For this review, take the finished solid that the model builds, in its own axes (mm). A direction names the side the tool comes from. Round coordinates to 2 decimals unless told otherwise and drop trailing zeros. Write each loop counter-clockwise with the first axis right and the second up, starting at its lowest first coordinate (ties: lowest second). Pieces come first, ordered by that corner, then holes. Notation, with made-up numbers: M 50,-22 L 80,-22 A29 ccw 80,4 Z; hole C -9.75,-15.75 d4. An arc over 180 degrees is marked long. Use one line per item in the form item = value. Start each with the question number.
Item 1: Add section A-A (x = 5.5). State the section outline as (y, z) points.
Item 2: For P1, Ø8.5, axis at x = -5, z = 4, coming from the +Y side; P2, Ø3, axis at y = 4.5, z = 3, coming from the +X side; P3, Ø3, axis at x = -8, z = -6, coming from the +Y side, all flat-tipped, find the tip position at first contact; note any pin that passes through.
Item 3: Draft analysis for pull direction Z (two halves, no side actions). For faces 1 (the conical face through (1.35, 3.288, 1.375)), 2 (the flat face through (5, 0.5, -4)), 3 (the flat face through (0, 0, 0)), 4 (the conical face through (-10.4, 3, 8.3)), state which applies: released by +Z, released by -Z, zero draft, split by the parting line, or undercut.
Item 4: Add section B-B (z = 4). State the section outline as (x, y) points, and give its area (3 significant figures).
Item 5: For line 1 (Z direction, x = 5.75, y = 1.25); line 2 (X direction, y = 1, z = 5.5); line 3 (Y direction, x = -9, z = -7), list the stretches that pass through material, from the lowest coordinate up. Write a range as [from, to].
Item 6: For faces 5 (the conical face through (10.21, 0.99, 8.23)), 6 (the conical face through (10.3, 3, 8.4)), 7 (the flat face through (10.704, 2.986, -0.105)), 8 (the conical face through (-10.23, 0.99, 8.21)), 9 (the conical face through (-0.218, 3.288, -1.663)), list the 3-axis set-ups (+Z, -Z, +X, -X, +Y, -Y) from which the entire face can be reached by the end or side of a thin tool; tool diameter is ignored.
from build123d import *

# Parameters (mm, degrees)
BOSS_EXTRUDE1_DEPTH = 4
BOSS_EXTRUDE1_DRAFT = -1
SHELL1_T            = -0.5
SKETCH2_R           = 2
BOSS_EXTRUDE2_DEPTH = 5.5
BOSS_EXTRUDE2_TAPER = 1.5
CIRPATTERN1_COUNT   = 4
SKETCH4_R           = 1.605977431
CUT_EXTRUDE1_DEPTH  = 5.5
CUT_EXTRUDE1_DRAFT  = 1.5
RIB2_START          = -10.069744096
RIB2_DEPTH          = 8.231928651
RIB2_START_2        = 1.837815445
RIB2_2_DEPTH        = 8.231928651
RIB2_START_3        = -8.069744096
RIB2_3_DEPTH        = 6.231928651
RIB2_4_DEPTH        = 6.231928651


with BuildPart() as part:
    # Sketch1 → Boss-Extrude1 (with draft: the straight prism first)
    with BuildSketch(Plane(origin=(0, 0, 0), x_dir=(1, 0, 0), z_dir=(0, 1, 0))):
        with BuildLine():
            Line((-9.5, -8.5), (9.5, -8.5))
            ThreePointArc((9.5, -8.5), (10.207106781, -8.207106781), (10.5, -7.5))
            Line((10.5, -7.5), (10.5, 7.5))
            ThreePointArc((10.5, 7.5), (10.207106781, 8.207106781), (9.5, 8.5))
            Line((9.5, 8.5), (-9.5, 8.5))
            ThreePointArc((-9.5, 8.5), (-10.207106781, 8.207106781), (-10.5, 7.5))
            Line((-10.5, 7.5), (-10.5, -7.5))
            ThreePointArc((-10.5, -7.5), (-10.207106781, -8.207106781), (-9.5, -8.5))
        make_face()
    extrude(amount=BOSS_EXTRUDE1_DEPTH)
    # Boss-Extrude1: the draft: its side faces are tilted about the plane it starts from
    boss_extrude1_sides = [part.faces().sort_by_distance(p)[0] for p in [
        (0, 2, 8.5),
        (10.207106781, 2, 8.207106781),
        (10.5, 2, 0),
        (10.207106781, 2, -8.207106781),
        (0, 2, -8.5),
        (-10.207106781, 2, -8.207106781),
        (-10.5, 2, 0),
        (-10.207106781, 2, 8.207106781),
    ]]
    draft(boss_extrude1_sides, Plane(origin=(0, 0, 0), x_dir=(1, 0, 0), z_dir=(0, 1, 0)), BOSS_EXTRUDE1_DRAFT)

    # Shell1
    shell1_openings = [part.faces().sort_by_distance(p)[0] for p in [
        (0, 4, 0),
    ]]
    offset(amount=SHELL1_T, openings=shell1_openings, kind=Kind.INTERSECTION)

    # Sketch2 → Boss-Extrude2 (add)
    with BuildSketch(Plane(origin=(0, 0.5, 0), x_dir=(1, 0, 0), z_dir=(0, 1, 0))):
        Circle(SKETCH2_R)
    extrude(amount=BOSS_EXTRUDE2_DEPTH, taper=BOSS_EXTRUDE2_TAPER)

    # Rib1: read off the stored shape, not the designer's step
    # Rib1: loft between two sections, ruled curve by curve
    rib1_from = [
        Edge.make_line((1.837815545, 6, 0.259010132), (2.355977431, 6, 0.25)),
        Edge.make_line((1.837815545, 6, -0.259010132), (2.355977431, 6, -0.25)),
        Edge.make_line((2.355977431, 6, -0.25), (2.355977431, 6, 0.25)),
        Edge.make_line((1.837815545, 6, -0.259010132), (1.837815545, 6, 0.259010132)),
    ]
    rib1_to = [
        Edge.make_line((1.982384256, 0.5, 0.264863479), (2.837165081, 0.5, 0.25)),
        Edge.make_line((1.982384256, 0.5, -0.264863479), (2.837165081, 0.5, -0.25)),
        Edge.make_line((2.837165081, 0.5, -0.25), (2.837165081, 0.5, 0.25)),
        Edge.make_line((1.982384256, 0.5, -0.264863479), (1.982384256, 0.5, 0.264863479)),
    ]
    rib1 = Solid(Shell([*[Face.make_surface_from_curves(rib1_from[k], rib1_to[k]) for k in range(4)], Face(Wire(rib1_from)), Face(Wire(rib1_to))]))
    add(rib1)

    # CirPattern1: Rib1 ×4 about axis
    cirpattern1_axis = Axis((0, 0, 0), (0, 1, 0))
    for i in range(1, CIRPATTERN1_COUNT):
        add(rib1.rotate(cirpattern1_axis, i * 360 / CIRPATTERN1_COUNT))


with BuildPart() as cut_extrude1_tool:
    # Sketch4 → Cut-Extrude1 (with draft: the straight prism first)
    with BuildSketch(Plane(origin=(0, 6, 0), x_dir=(1, 0, 0), z_dir=(0, 1, 0))):
        Circle(SKETCH4_R)
    extrude(amount=-CUT_EXTRUDE1_DEPTH)
    # Cut-Extrude1: the draft: its side faces are tilted about the plane it starts from
    cut_extrude1_sides = [cut_extrude1_tool.faces().sort_by_distance(p)[0] for p in [
        (-1.605977431, 3.25, 0),
    ]]
    draft(cut_extrude1_sides, Plane(origin=(0, 6, 0), x_dir=(1, 0, 0), z_dir=(0, 1, 0)), CUT_EXTRUDE1_DRAFT)


with BuildPart() as part_1:
    add(part.part)

    # Cut-Extrude1: cut by cut_extrude1_tool
    add(cut_extrude1_tool.part, mode=Mode.SUBTRACT)

    # Sweep1: sweep along a path in Sketch6
    with BuildLine(Plane(origin=(0, 2, 0), x_dir=(-1, 0, 0), z_dir=(0, -1, 0))) as sweep1_path:
        Line((-9.5, 8.56982026), (9.5, 8.56982026))
        ThreePointArc((9.5, 8.56982026), (10.25647716, 8.25647716), (10.56982026, 7.5))
        Line((10.56982026, 7.5), (10.56982026, -7.5))
        ThreePointArc((10.56982026, -7.5), (10.25647716, -8.25647716), (9.5, -8.56982026))
        Line((9.5, -8.56982026), (-9.5, -8.56982026))
        ThreePointArc((-9.5, -8.56982026), (-10.25647716, -8.25647716), (-10.56982026, -7.5))
        Line((-10.56982026, -7.5), (-10.56982026, 7.5))
        ThreePointArc((-10.56982026, 7.5), (-10.25647716, 8.25647716), (-9.5, 8.56982026))
    # Sketch5 → Sweep1 (sweep)
    with BuildSketch(Plane.XY):
        Polygon((10.56982026, 4), (10.53491013, 2), (10.83491013, 2), align=None)
    sweep(path=sweep1_path.line)

    # Rib2: read off the stored shape, not the designer's step
    # Rib2 outline → Rib2 (add)
    with BuildSketch(Plane.YZ.offset(RIB2_START)):
        Polygon((2, 0.25), (0.5, 0.276182597), (0.5, -0.276182597), (2, -0.25), align=None)
    extrude(amount=RIB2_DEPTH)

    # Rib2 2 outline → Rib2 2 (add)
    with BuildSketch(Plane.YZ.offset(RIB2_START_2)):
        Polygon((2, 0.25), (0.5, 0.276182597), (0.5, -0.276182597), (2, -0.25), align=None)
    extrude(amount=RIB2_2_DEPTH)

    # Rib2 3 outline → Rib2 3 (add)
    with BuildSketch(Plane.XY.offset(RIB2_START_3)):
        Polygon((0.276182597, 0.5), (0.25, 2), (-0.25, 2), (-0.276182597, 0.5), align=None)
    extrude(amount=RIB2_3_DEPTH)

    # Rib2 4 outline → Rib2 4 (add)
    with BuildSketch(Plane.XY.offset(RIB2_START_2)):
        Polygon((0.276182597, 0.5), (0.25, 2), (-0.25, 2), (-0.276182597, 0.5), align=None)
    extrude(amount=RIB2_4_DEPTH)


solid = part_1.part
Calculated:
q1.outline = M 0,-8.5 L 2,-8.53 L 2,-8.83 L 4,-8.57 L 4,-8.07 L 0.5,-8.01 L 0.5,-0.28 L 2,-0.25 L 2,0.25 L 0.5,0.28 L 0.5,8.01 L 4,8.07 L 4,8.57 L 2,8.83 L 2,8.53 L 0,8.5 Z
q2.P1 = 4
q2.P2 = 10.7
q2.P3 = 0.5
q3.face_1 = undercut
q3.face_2 = undercut
q3.face_3 = zero draft
q3.face_4 = released by +Z
q4.outline = M -10.83,2 L -10.53,2 L -10.5,0 L 10.5,0 L 10.53,2 L 10.83,2 L 10.57,4 L 10.07,4 L 10.01,0.5 L 0.28,0.5 L 0.25,2 L -0.25,2 L -0.28,0.5 L -10.01,0.5 L -10.07,4 L -10.57,4 Z
q4.area = 15.4 mm^2
q5.line_1 = [-8.52, -8.02], [-0.26, 0.26], [8.02, 8.52]
q5.line_2 = [-10.52, -10.02], [-0.27, 0.27], [10.02, 10.52]
q5.line_3 = [0, 0.5]
q6.face_5 = +Z, +X, -Y
q6.face_6 = +Z, +X, +Y
q6.face_7 = +Z, -Z, +X, +Y
q6.face_8 = +Z, -X, -Y
q6.face_9 = none
